Answer from the drawing. Dimensions are ordinates in mm from the lowest x, y and z of the part. A direction names the side the tool comes from. Round coordinates to 2 decimals unless told otherwise and drop trailing zeros. Write each loop counter-clockwise with the first axis right and the second up, starting at its lowest first coordinate (ties: lowest second). Pieces come first, ordered by that corner, then holes. Notation, with made-up numbers: (5, -39) -> (53, -39) arc R17 ccw to (53, -11) -> close; hole circle Ø4 at (85.25, 64.5). An arc over 180 degrees is marked (long way). Return JSON: item names as keys, results as strings. Group by question number.
(1) A cutting plane is placed at A-A on z = 25.5. Give the vertices of the cut face in (x, y).
(2) The mould has two halves that part along X. Classify the marked faces 1, 2, 3 and 4: released by +X, released by -X, zero draft, split by the parting line, or undercut.
(3) A cutting plane is placed at C-C on y = 31.5. Give the vertices of the cut face in (x, z), then the cut area to 3 significant figures.
(4) A cutting plane is placed at B-B on x = 33. Give the vertices of the cut face in (y, z).
(5) A cutting plane is placed at D-D on y = 43. Give the vertices of the cut face in (x, z).
(6) For the marked faces 5 and 6, determine the directions among +Z, -Z, +X, -X, +Y, -Y from which every point of the face is accessible in a straight line to the end or side of a thin tool.
(7) Straight lines are drawn through the part: line 1 (X direction, y = 7.5, z = 18); line 2 (Z direction, x = 86, y = 3.5); line 3 (Z direction, x = 62, y = 27). For each, find the intervals that lie inside material, in ascending order.
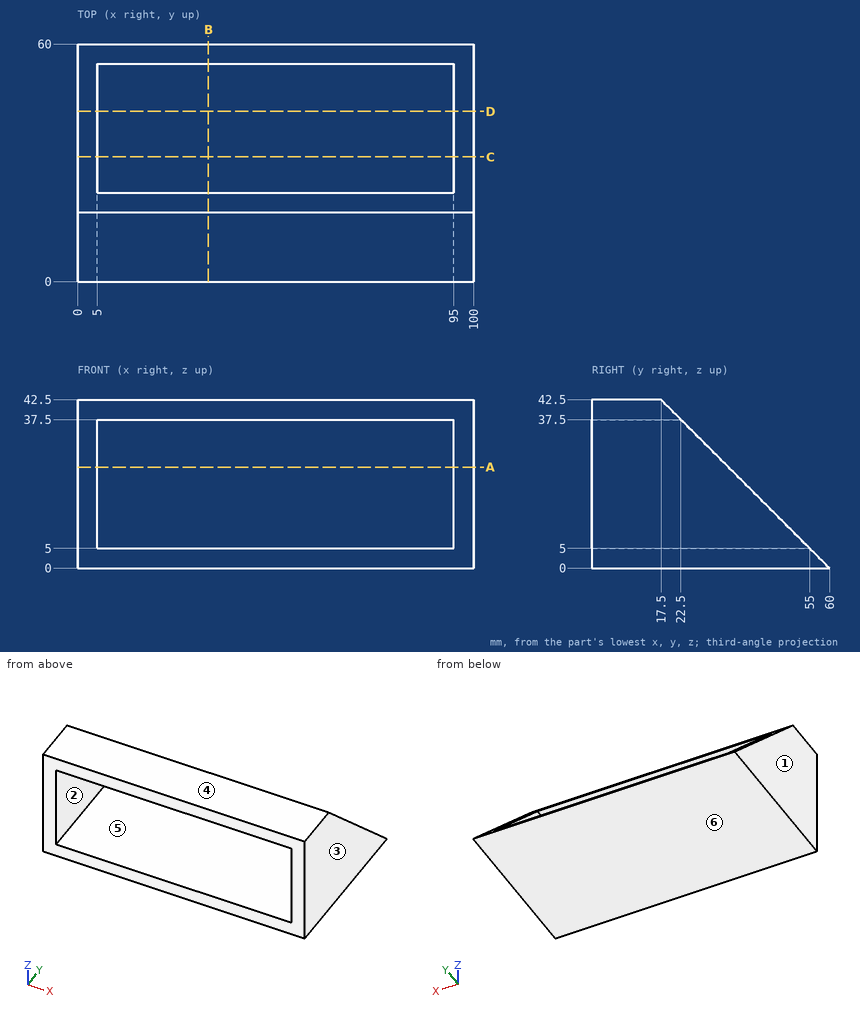
Checks:
{
 "1": {"outline": "(0, 0) -> (5, 0) -> (5, 34.5) -> (0, 34.5) -> close; (95, 0) -> (100, 0) -> (100, 34.5) -> (95, 34.5) -> close"},
 "2": {"face 1": "released by -X", "face 2": "undercut", "face 3": "released by +X", "face 4": "zero draft"},
 "3": {"outline": "(0, 0) -> (100, 0) -> (100, 28.5) -> (95, 28.5) -> (95, 5) -> (5, 5) -> (5, 28.5) -> (0, 28.5) -> close", "area": "735 mm^2"},
 "4": {"outline": "(0, 0) -> (60, 0) -> (55, 5) -> (0, 5) -> close; (0, 37.5) -> (22.5, 37.5) -> (17.5, 42.5) -> (0, 42.5) -> close"},
 "5": {"outline": "(0, 0) -> (100, 0) -> (100, 17) -> (95, 17) -> (95, 5) -> (5, 5) -> (5, 17) -> (0, 17) -> close"},
 "6": {"face 5": "+Y, -Y", "face 6": "-Z, +X, -X, +Y, -Y"},
 "7": {"line 1": "x = 0 to 5, 95 to 100", "line 2": "z = 0 to 5, 37.5 to 42.5", "line 3": "z = 0 to 5"}
}
